```python
from build123d import *

# Parameters (mm, degrees)
F0_R     = 20
F0_R_2   = 15.07
F1_DEPTH = 10.8
F2_R     = 13.5
F3_DEPTH = 10.8
F4_R     = 20
F4_R_2   = 15.07
F5_DEPTH = 14.4
F6_R     = 20
F6_R_2   = 15.7
F7_DEPTH = 1.3
F8_R     = 20
F8_R_2   = 15.7
F8_R_3   = 15.07
F9_DEPTH = 9.5


with BuildPart() as f1:
    # F0 (on Front) → F1 (new body)
    with BuildSketch(Plane.XZ):
        Circle(F0_R)
        Circle(F0_R_2, mode=Mode.SUBTRACT)
        Circle(F0_R_2)
    extrude(amount=F1_DEPTH)

    # F2 (on face) → F3 (cut)
    with BuildSketch(Plane(origin=(0, 0, 0), x_dir=(-1, 0, 0), z_dir=(0, 1, 0))):
        Circle(F2_R)
    extrude(amount=-F3_DEPTH, mode=Mode.SUBTRACT)

    # F4 (on face) → F5 (join)
    with BuildSketch(Plane.XZ.offset(10.8)):
        Circle(F4_R)
        Circle(F4_R_2, mode=Mode.SUBTRACT)
    extrude(amount=F5_DEPTH)

    # F6 (on face) → F7 (join)
    with BuildSketch(Plane.XZ.offset(25.2)):
        Circle(F6_R)
        Circle(F6_R_2, mode=Mode.SUBTRACT)
    extrude(amount=F7_DEPTH)

    # F8 (on face) → F9 (join)
    with BuildSketch(Plane.XZ.offset(26.5)):
        Circle(F8_R)
        Circle(F8_R_2, mode=Mode.SUBTRACT)
        Circle(F8_R_2)
        Circle(F8_R_3, mode=Mode.SUBTRACT)
    extrude(amount=F9_DEPTH)


solid = f1.part
```
Geometry check sheet. Reference: the model listing, model coordinates, mm. A direction names the side the tool comes from. Coordinates: 2 decimals unless noted, no trailing zeros. Write each loop counter-clockwise with the first axis right and the second up, starting at its lowest first coordinate (ties: lowest second). Pieces come first, ordered by that corner, then holes. Notation, with made-up numbers: M -14.75,32 L 39.25,32 A16 ccw 39.25,51 Z; hole C 59,-14.75 d1. An arc over 180 degrees is marked long. Answer as a JSON object with one key per item and string values.
1. Section check D-D, the plane x = 17. Enter the section's corners in (y, z).
Answers below:
{"outline": "M -36,-10.54 L 0,-10.54 L 0,10.54 L -36,10.54 Z"}
2. Section check B-B, the plane z = 0. Enter the section's corners in (x, y).
Answers below:
{"outline": "M -20,-36 L -15.07,-36 L -15.07,-26.5 L -15.7,-26.5 L -15.7,-25.2 L -15.07,-25.2 L -15.07,-10.8 L -13.5,-10.8 L -13.5,0 L -20,0 Z; M 13.5,-10.8 L 15.07,-10.8 L 15.07,-25.2 L 15.7,-25.2 L 15.7,-26.5 L 15.07,-26.5 L 15.07,-36 L 20,-36 L 20,0 L 13.5,0 Z"}
3. Go/stop test with flat-tipped pins: pin 1 Ø3 at (y, z) = (-12.5, -8.5) entering from -X (3 decimals); pin 2 Ø10 at (x, y) = (2, -22) entering from -Z; pin 3 Ø4 at (x, y) = (-10.5, -20) entering from -Z; pin 4 Ø24 at (x, z) = (0, 0) entering from +Y. Record where each tip stops, or that it passes through.
Answers below:
{"pin 1": "stops at x = -18.735", "pin 2": "stops at z = -20", "pin 3": "stops at z = -18.1", "pin 4": "passes through"}
4. Draft check along X on faces 1 (the cylindrical face through (-3.27, -17.9, -14.71)), 2 (the flat face through (3, -36, 15)), 3 (the cylindrical face through (-4.336, -17.748, -19.524)). Enter one of: released by +X, released by -X, zero draft, split by the parting line, or undercut.
Answers below:
{"face 1": "undercut", "face 2": "zero draft", "face 3": "split by the parting line"}
5. Section check A-A, the plane x = 0. Enter the section's corners in (y, z), plus the area to 3 significant figures.
Answers below:
{"outline": "M -36,-20 L 0,-20 L 0,-13.5 L -10.8,-13.5 L -10.8,-15.07 L -25.2,-15.07 L -25.2,-15.7 L -26.5,-15.7 L -26.5,-15.07 L -36,-15.07 Z; M -36,15.07 L -26.5,15.07 L -26.5,15.7 L -25.2,15.7 L -25.2,15.07 L -10.8,15.07 L -10.8,13.5 L 0,13.5 L 0,20 L -36,20 Z", "area": "387 mm²"}
6. Tool access check on faces 4 (the flat face through (-6, -25.2, 14)), 5 (the flat face through (-13.5, -10.8, 2.3)), 6 (the flat face through (13.1, 0, -4.2)). Record the directions out of +Z, -Z, +X, -X, +Y, -Y that give a thin tool (end or side, any length) a straight path to the whole face; none if there is none.
Answers below:
{"face 4": "none", "face 5": "-Y", "face 6": "+Z, -Z, +X, -X, +Y"}
7. Scan lines: L1, parallel to Z at x = 0, y = -3; L2, parallel to Z at x = 0, y = -34; L3, parallel to Y at x = -15.5, z = 1. Record each from-to range of solid material in increasing order.
Answers below:
{"L1": "z = -20 to -13.5, 13.5 to 20", "L2": "z = -20 to -15.07, 15.07 to 20", "L3": "y = -36 to -26.5, -25.2 to 0"}
8. Section check C-C, the plane y = -1.5. Enter the section's corners in (x, z), plus the area to 3 significant figures.
Answers below:
{"outline": "C 0,0 d40; hole C 0,0 d27", "area": "684 mm²"}
